```python
from build123d import *

# Parameters (mm, degrees)
POCKET_DEPTH      = 22.501
POCKET_DEPTH_BACK = -22.501


with BuildPart() as part:
    # Sketch → Revolution (revolve)
    with BuildSketch(Plane.XZ):
        Polygon((-22.5, 0), (-15.5, 0), (-15.5, 75), (-4.1, 93.15), (-4.1, 102.15), (-5.1, 103.15), (-8.1, 103.15), (-13, 107.35), (-13, 119.15), (-16, 122.15), (-22.5, 122.15), align=None)
    revolve(axis=Axis((0, 0, 0), (0, 0, 1)))

    # Sketch001 → Pocket (cut, two sides)
    with BuildSketch(Plane.XZ) as pocket_sk:
        with BuildLine():
            ThreePointArc((-10, 23), (0, 13), (10, 23))
            Line((10, 23), (10, 43))
            ThreePointArc((10, 43), (0, 53), (-10, 43))
            Line((-10, 43), (-10, 23))
        make_face()
    extrude(amount=-POCKET_DEPTH, mode=Mode.SUBTRACT)
    extrude(pocket_sk.sketch, amount=-POCKET_DEPTH_BACK, mode=Mode.SUBTRACT)


solid = part.part
```
Design review of the part built by this model. Coordinates are the model's own, in mm. A direction names the side the tool comes from. Give positions to 0.01 mm unless a question says otherwise; leave off trailing zeros. Write each loop counter-clockwise with the first axis right and the second up, starting at its lowest first coordinate (ties: lowest second). Pieces come first, ordered by that corner, then holes. Notation, with made-up numbers: (-26, 48) - (33, 48) arc R24 cw to (33, 87) - close; hole circle Ø5 at (76.5, 78.25). An arc over 180 degrees is marked (long way). Return JSON: item names as keys, results as strings. Group by question number.
(1) Mouldability with a two-part tool opening along X and no side actions: class faces 4 (the conical face through (5.7, 4.37, 88.24)), 5 (the cylindrical face through (-20.784, 8.618, 60.22)), 6 (the flat face through (5, 15, 0)) as +X half, -X half, draft (parallel to the pull), parting line (faces both ways), or undercut.
(2) We need section D-D, the plane z = 72.5. Give the boundary of the cut face in (x, y), then the cut area to 3 significant figures.
(3) To check wall thickness, follow probe 1 along Y at (x, z) = (0, 98.75); probe 2 along Y at (x, z) = (0, 112.75). State the ranges of each line that lie inside material, in increasing order.
(4) We need section C-C, the plane y = 0. Give the boundary of the cut face in (x, z).
(5) Machinability: for faces 1 (the cylindrical face through (15.485, -0.682, 38.025)), 2 (the flat face through (10, 16, 33)), 3 (the cylindrical face through (10.316, 7.91, 113.333)), which of the approach directions +Z, -Z, +X, -X, +Y, -Y give a long, thin tool a straight path to every point of the face, cutting with its end or side? Answer none if there is none.
(6) Insertion check: pin 1 (4 mm diameter, centred on y = 14.5, z = 32.5, fed in from -X); pin 2 (5 mm diameter, centred on y = 10.5, z = 83.5, fed in from +X); pin 3 (2 mm diameter, centred on x = -10, z = 13.5, fed in from -Y); pin 4 (12 mm diameter, centred on x = -15.5, y = 16, fed in from -Z). Each pin has a flat end and moves straight along its axis. Give the tip position at first contact, or say it passes through.
(7) We need section B-B, the plane z = 38. Give the boundary of the cut face in (x, y).
(8) We need section A-A, the plane x = 0. Give the number of separate pieces and of enclosed holes in the cut face, then the cut area to 3 significant figures.
Reported:
{
 "1": {"face 4": "undercut", "face 5": "parting line", "face 6": "draft"},
 "2": {"outline": "circle Ø45 at (0, 0); hole circle Ø31 at (0, 0)", "area": "836 mm2"},
 "3": {"probe 1": "y = -22.5 to -4.1, 4.1 to 22.5", "probe 2": "y = -22.5 to -13, 13 to 22.5"},
 "4": {"outline": "(-22.5, 0) - (-15.5, 0) - (-15.5, 75) - (-4.1, 93.15) - (-4.1, 102.15) - (-5.1, 103.15) - (-8.1, 103.15) - (-13, 107.35) - (-13, 119.15) - (-16, 122.15) - (-22.5, 122.15) - close; (4.1, 93.15) - (15.5, 75) - (15.5, 0) - (22.5, 0) - (22.5, 122.15) - (16, 122.15) - (13, 119.15) - (13, 107.35) - (8.1, 103.15) - (5.1, 103.15) - (4.1, 102.15) - close"},
 "5": {"face 1": "-Z", "face 2": "+Y, -Y", "face 3": "+Z"},
 "6": {"pin 1": "stops at x = -18.71", "pin 2": "stops at x = 21.03", "pin 3": "stops at y = -20.62", "pin 4": "stops at z = 0"},
 "7": {"outline": "(-10, -20.16) - (-10, -11.84) arc R15.5 cw to (-10, 11.84) - (-10, 20.16) arc R22.5 ccw to start; (10, -20.16) arc R22.5 ccw to (10, 20.16) - (10, 11.84) arc R15.5 cw to (10, -11.84) - close"},
 "8": {"separate pieces": "4", "enclosed holes": "0", "area": "1,690 mm2"}
}
